Verification items for this drawing (mm, ordinates from the low corner). A direction names the side the tool comes from. Coordinates: 2 decimals unless noted, no trailing zeros. Order: outer loops, then holes, each group sorted by start corner. A loop starts at its lowest first (then second) coordinate and runs counter-clockwise, first axis right, second up. Notation, with made-up numbers: (78, -19) -> (97, -19) arc R25 cw to (97, 14) -> close; hole circle Ø9 at (18.25, -30.5). An arc over 180 degrees is marked (long way). Write each question's results on one line, items separated by ' | '. Start each with the question number.
(1) Cross-section at A-A on z = 19. Enter the section's corners in (x, y), and give its area (3 significant figures).
(2) Go/stop test with flat-tipped pins: pin 1 (10 mm diameter, centred on x = 9, z = 29, fed in from +Y); pin 2 (1 mm diameter, centred on x = 14.5, z = 19, fed in from -Y); pin 3 (3 mm diameter, centred on x = 14, z = 14.5, fed in from +Y). Record where each tip stops, or that it passes through.
(3) Draft check along Y on the marked faces 4, 5 and 6. Enter one of: +Y half, -Y half, draft (parallel to the pull), parting line (faces both ways), or undercut.
(4) Set-up check for the marked faces 1, 2 and 3: record each of +Z, -Z, +X, -X, +Y, -Y from which the full face is reachable in a straight line by a thin tool's end or side.
(5) Thickness scan on probe 1 along Y at (x, z) = (12.5, 14); probe 2 along Y at (x, z) = (1.5, 17); probe 3 along Y at (x, z) = (13.75, 20.5). Record the ranges inside material, lowest first. Write a range as [from, to].
(6) Cross-section at D-D on z = 5. Enter the section's corners in (x, y), and give its area (3 significant figures).
(7) Cross-section at B-B on x = 10. Enter the section's corners in (y, z), and give its area (3 significant figures).
(8) Cross-section at C-C on x = 18.25. Enter the section's corners in (y, z), and give its area (3 significant figures).
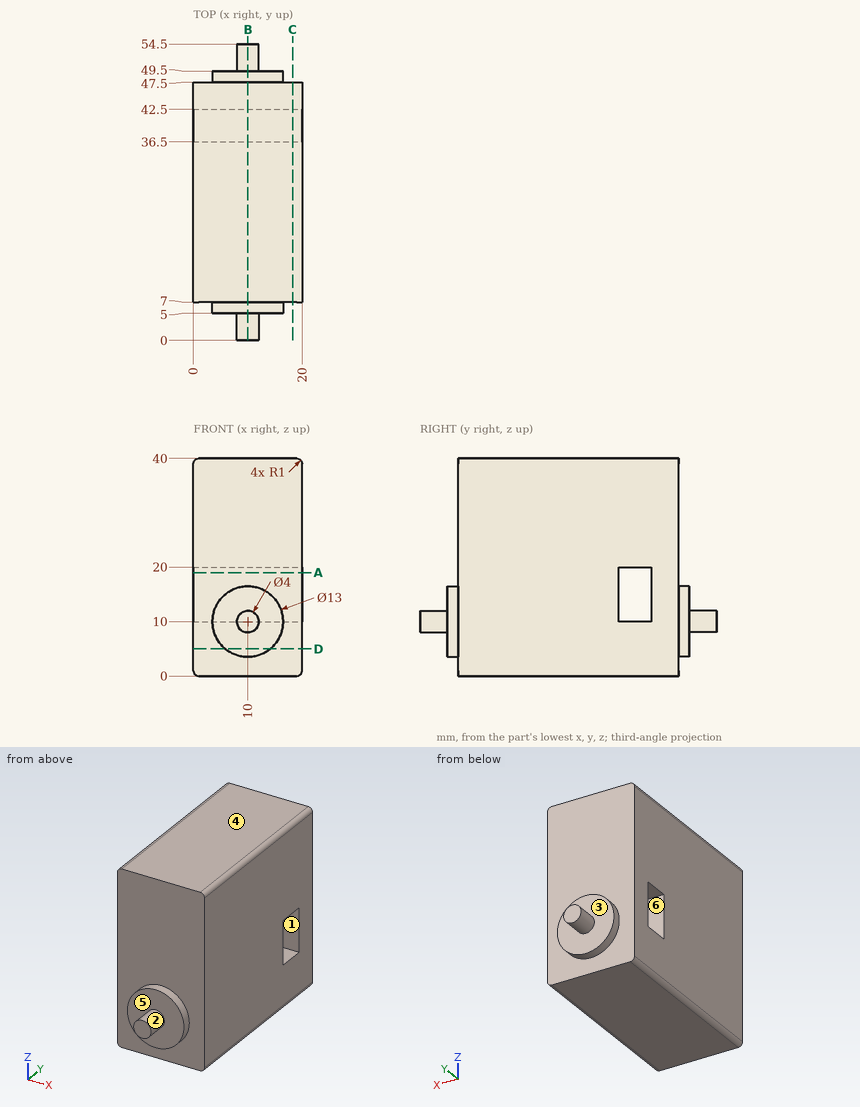
Results are:
1) outline: (0, 7) -> (20, 7) -> (20, 36.5) -> (0, 36.5) -> close; (0, 42.5) -> (20, 42.5) -> (20, 47.5) -> (0, 47.5) -> close | area: 690 mm2
2) pin 1: stops at y = 47.5 | pin 2: stops at y = 7 | pin 3: stops at y = 49.5
3) face 4: draft | face 5: -Y half | face 6: undercut
4) face 1: +X, -X | face 2: -Y | face 3: +Y
5) probe 1: y = [5, 36.5], [42.5, 49.5] | probe 2: y = [7, 36.5], [42.5, 47.5] | probe 3: y = [7, 47.5]
6) outline: (0, 7) -> (5.85, 7) -> (5.85, 5) -> (14.15, 5) -> (14.15, 7) -> (20, 7) -> (20, 47.5) -> (14.15, 47.5) -> (14.15, 49.5) -> (5.85, 49.5) -> (5.85, 47.5) -> (0, 47.5) -> close | area: 843 mm2
7) outline: (0, 8) -> (5, 8) -> (5, 3.5) -> (7, 3.5) -> (7, 0) -> (47.5, 0) -> (47.5, 3.5) -> (49.5, 3.5) -> (49.5, 8) -> (54.5, 8) -> (54.5, 12) -> (49.5, 12) -> (49.5, 16.5) -> (47.5, 16.5) -> (47.5, 40) -> (7, 40) -> (7, 16.5) -> (5, 16.5) -> (5, 12) -> (0, 12) -> close; hole (36.5, 10) -> (42.5, 10) -> (42.5, 20) -> (36.5, 20) -> close | area: 1,650 mm2
8) outline: (7, 0) -> (47.5, 0) -> (47.5, 40) -> (7, 40) -> close; hole (36.5, 10) -> (42.5, 10) -> (42.5, 20) -> (36.5, 20) -> close | area: 1,560 mm2
